from build123d import *

# Parameters (mm, degrees)
SKETCH_1_R      = 2
EXTRUDE_1_DEPTH = 3


with BuildPart() as part:
    # 草图1 → 凸台-拉伸1 (new body)
    with BuildSketch(Plane.XY):
        with BuildLine():
            Line((254.002581869, 28.707860978), (294.002581869, 53.707860978))
            Line((294.002581869, 53.707860978), (294.002581869, 13.707860978))
            Line((294.002581869, 13.707860978), (294.002581869, -26.292139022))
            Line((294.002581869, -26.292139022), (254.002581869, -1.292139022))
            ThreePointArc((254.002581869, -1.292139022), (239.002581869, 13.707860978), (254.002581869, 28.707860978))
        make_face()
        with Locations((254.002581869, 13.707860978)):
            Circle(SKETCH_1_R, mode=Mode.SUBTRACT)
    extrude(amount=EXTRUDE_1_DEPTH)


solid = part.part
Input: part model. Units: mm. Frame: model coordinates. Coordinates: 2 decimals unless noted, no trailing zeros. Order: outer loops, then holes, each group sorted by start corner. A loop starts at its lowest first (then second) coordinate and runs counter-clockwise, first axis right, second up. Notation, with made-up numbers: M 42.5,12.25 L 69.5,12.25 A17 cw 69.5,24.25 Z; hole C 15,51.5 d6. An arc over 180 degrees is marked long. Answer in a Markdown table with one row per item.
(1) Section query A-A, the plane z = 0.9. Output: boundary loops of the cut face in (x, y), plus the area to 3 significant figures.
Numbers:
| item | result |
|---|---|
| outline | M 254,-1.29 L 294,-26.29 L 294,53.71 L 254,28.71 A15 ccw Z; hole C 254,13.71 d4 |
| area | 2,540 mm^2 |
(2) Contact query for a flat-ended pin moving along its axis: pin 1 Ø1 at (x, z) = (262, 1) entering from -Y. Output: stop coordinate, or through.
Numbers:
| item | result |
|---|---|
| pin 1 | stops at y = -6.6 |
(3) Section query B-B, the plane y = 41. Output: boundary loops of the cut face in (x, z), plus the area to 3 significant figures.
Numbers:
| item | result |
|---|---|
| outline | M 273.67,0 L 294,0 L 294,3 L 273.67,3 Z |
| area | 61.0 mm^2 |
(4) Material intervals for line 1 (Y direction, x = 252.5, z = 0.8); line 2 (Y direction, x = 254.5, z = 2); line 3 (X direction, y = 2.5, z = 0.25), sorted ascending. Write a range as [from, to].
Numbers:
| item | result |
|---|---|
| line 1 | y = [-1.22, 12.39], [15.03, 28.63] |
| line 2 | y = [-1.6, 11.77], [15.65, 29.02] |
| line 3 | x = [244.03, 294] |
(5) Section query C-C, the plane x = 262. Output: boundary loops of the cut face in (y, z).
Numbers:
| item | result |
|---|---|
| outline | M -6.29,0 L 33.71,0 L 33.71,3 L -6.29,3 Z |
(6) Draft query along Y for faces 1 (the flat face through (274.283, -13.967, 1.479)), 2 (the cylindrical face through (255.85, 12.94, 1.48)), 3 (the flat face through (273.72, 41.03, 1.48)), 4 (the flat face through (273, 14, 0)). Return one class per face: pulls with the +Y half, pulls with the -Y half, needs draft (parallel to the pull), parting line crosses it, or undercut.
Numbers:
| item | result |
|---|---|
| face 1 | pulls with the -Y half |
| face 2 | undercut |
| face 3 | pulls with the +Y half |
| face 4 | needs draft |
